Geometry: final body of the model. Coordinates: model frame, mm. Face numbers are marked on the shaded views. A direction names the side the tool comes from. Give positions to 0.01 mm unless a question says otherwise; leave off trailing zeros. Loops run counter-clockwise (first coordinate to the right, second up) from the corner with the lowest first, then second, coordinate; pieces in that order, holes last. Notation, with made-up numbers: (58.5, 20.25) -> (83.5, 20.25) arc R18 cw to (83.5, 38.25) -> close; hole circle Ø9 at (-37, 89.5). An arc over 180 degrees is marked (long way). Answer in a Markdown table with one row per item. Add a question column.
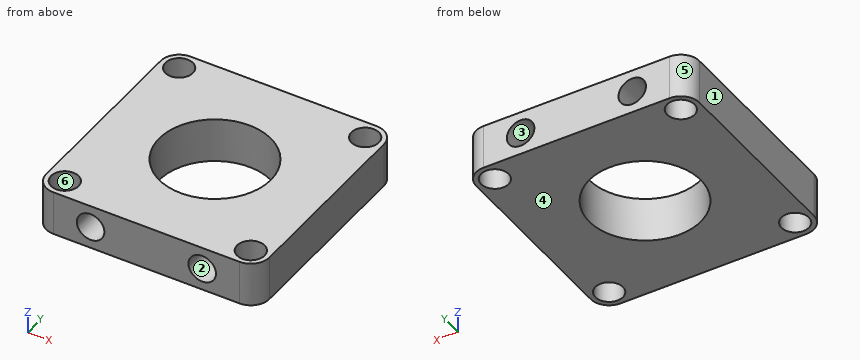
Autodesk Inventor part; units mm, degrees
ref_plane "YZ Plane" through (0, 0, 0) normal (1, 0, 0) x (0, 1, 0)
ref_plane "XZ Plane" through (0, 0, 0) normal (0, 1, 0) x (-1, 0, 0)
ref_plane "XY Plane" through (0, 0, 0) normal (0, 0, 1) x (1, 0, 0)
sketch "Sketch1" plane through (0, 0, 0) normal (0, 0, 1) x (1, 0, 0)
  line L0 (0, 0) -> (38.1, 0)
  line L1 (38.1, 0) -> (38.1, 38.1)
  line L2 (38.1, 38.1) -> (0, 38.1)
  line L3 (0, 38.1) -> (0, 0)
  circle A0 centre (3.175, 34.925) radius 2.3495
  circle A1 centre (34.925, 34.925) radius 2.3495
  circle A2 centre (3.175, 3.175) radius 2.3495
  circle A3 centre (34.925, 3.175) radius 2.3495
  line L4 (0, 19.05) -> (19.05, 19.05)
  circle A4 centre (19.05, 19.05) radius 9.525
  circle A5 centre (19.05, 19.05) radius 6.35
  line L5 (7.4295, 34.925) -> (7.4295, 38.1)
  line L6 (0, 30.6705) -> (3.175, 30.6705)
  arc A6 (3.175, 30.6705) -> (7.4295, 34.925) centre (3.175, 34.925) ccw
  line L7 (5.5245, 34.925) -> (7.4295, 34.925)
  line L8 (3.175, 7.4295) -> (0, 7.4295)
  line L9 (7.4295, 0) -> (7.4295, 3.175)
  arc A7 (7.4295, 3.175) -> (3.175, 7.4295) centre (3.175, 3.175) ccw
  line L10 (30.6705, 3.175) -> (30.6705, 0)
  line L11 (38.1, 7.4295) -> (34.925, 7.4295)
  arc A8 (34.925, 7.4295) -> (30.6705, 3.175) centre (34.925, 3.175) ccw
  line L12 (34.925, 30.6705) -> (38.1, 30.6705)
  line L13 (30.6705, 38.1) -> (30.6705, 34.925)
  arc A9 (30.6705, 34.925) -> (34.925, 30.6705) centre (34.925, 34.925) ccw
  line L14 (0, 7.4295) -> (0, 0)
  line L15 (0, 0) -> (7.4295, 0)
  line L16 (30.6705, 0) -> (38.1, 0)
  line L17 (38.1, 0) -> (38.1, 7.4295)
  line L18 (30.6705, 38.1) -> (38.1, 38.1)
  line L19 (38.1, 38.1) -> (38.1, 30.6705)
  dimension "d2" = 4.699
  dimension "d0" = 38.1
  dimension "d1" = 38.1
  dimension "d5" = 31.75
  dimension "d8" = 31.75
  dimension "d11" = 3.175
  dimension "d12" = 3.175
  dimension "d13" = 19.05
  dimension "d14" = 19.05
  dimension "d15" = 12.7
  dimension "d16" = 3.175
  dimension "d17" = 3.175
  dimension "d18" = 1.905
  dimension "d24" = 360
extrude "Extrusion1" add sketch "Sketch1" along normal blind 7.62 contours L3 L8 A7 L9 L0 | L9 A7 L8 L3 L6 A6 L5 L2 L13 A9 L12 L1 L11 A8 L10 L0 | L10 A8 L11 L1 L0 | L3 L2 L5 A6 L6 | L12 A9 L13 L2 L1
fillet "Fillet1" radius 3.175 4 edges at (0, 38.1, 3.81) (38.1, 38.1, 3.81) (0, 0, 3.81) (38.1, 0, 3.81)
sketch "Sketch2" plane through (3.175, 38.1, 0) normal (0, 1, 0) x (1, 0, 0)
  line L0 (31.75, 0) -> (0, 0)
  line L1 (0, -7.62) -> (31.75, -7.62)
  line L2 (15.875, 0) -> (15.875, -3.81)
  line L3 (15.875, -3.81) -> (25.4, -3.81)
  line L4 (15.875, -3.81) -> (6.35, -3.81)
  circle A0 centre (25.4, -3.81) radius 2.3495
  circle A1 centre (6.35, -3.81) radius 2.3495
  point P0 (-3.175, 0)
  dimension "d29" = 3.81
  dimension "d30" = 9.525
  dimension "d31" = 9.525
  dimension "d32" = 4.699
  dimension "d33" = 4.699
extrude "Extrusion2" cut sketch "Sketch2" against normal blind 7.62
sketch "Sketch3" plane through (3.175, 0, 0) normal (0, -1, 0) x (1, 0, 0)
  line L0 (0, 0) -> (31.75, 0)
  line L1 (15.875, 0) -> (15.875, 3.81)
  line L2 (15.875, 3.81) -> (6.35, 3.81)
  line L3 (15.875, 3.81) -> (25.4, 3.81)
  circle A0 centre (6.35, 3.81) radius 2.3495
  circle A1 centre (25.4, 3.81) radius 2.3495
  point P0 (-3.175, 0)
  dimension "d36" = 3.81
  dimension "d37" = 9.525
  dimension "d38" = 9.525
  dimension "d39" = 4.699
  dimension "d40" = 4.699
extrude "Extrusion3" cut sketch "Sketch3" against normal blind 7.62
thread "Thread1"
thread "Thread2"
thread "Thread3"
thread "Thread4"
thread "Thread5"
thread "Thread6"
thread "Thread7"
thread "Thread8"
equation "\"d16\" = d11"
equation "\"d17\" = d11"
properties part number "Gearbox End Plate 2"
(1) Cut plane B-B on y = 4. Return the cut outline in (x, z) (1 decimal).
(2) Cut plane D-D on z = 3.81. State how many separate pieces and enclosed holes the cut face has, then the cut area to 3 significant figures.
(3) Pin query (flat end, axial travel): pin 1 Ø2.5 at (x, z) = (29, 4) entering from -Y; pin 2 Ø2.5 at (x, z) = (9, 4.5) entering from +Y. Return the tip coordinate at first contact, or that it passes through.
(4) Cut plane A-A on x = 19.05. Return the cut outline in (y, z) (3 decimals).
(5) Draft query along X for the marked faces 4, 5 and 6. Return one class per face: +X half, -X half, draft (parallel to the pull), parting line (faces both ways), or undercut.
(6) Material intervals for line 1 along X through (y, z) = (34.75, 3.81); line 2 along Y through (x, z) = (3, 1.25); line 3 along Y through (x, z) = (33, 5.5), sorted ascending. Write a range as from..to.
(7) Reachability of the marked faces 1, 2 and 3 from +Z, -Z, +X, -X, +Y, -Y: full face, straight path, thin tool, end or side. Return the list, or none.
Answer list:
| question | item | result |
|---|---|---|
| 1 | outline | (0, 0) -> (1, 0) -> (1, 7.6) -> (0, 7.6) -> close; (5.4, 0) -> (32.7, 0) -> (32.7, 7.6) -> (5.4, 7.6) -> close; (37.1, 0) -> (38.1, 0) -> (38.1, 7.6) -> (37.1, 7.6) -> close; hole circle Ø4.7 at (9.5, 3.8); hole circle Ø4.7 at (28.6, 3.8) |
| 2 | separate pieces | 1 |
| 2 | enclosed holes | 5 |
| 2 | area | 945 mm² |
| 3 | pin 1 | stops at y = 7.62 |
| 3 | pin 2 | stops at y = 30.48 |
| 4 | outline | (0, 0) -> (9.525, 0) -> (9.525, 7.62) -> (0, 7.62) -> close; (28.575, 0) -> (38.1, 0) -> (38.1, 7.62) -> (28.575, 7.62) -> close |
| 5 | face 4 | draft |
| 5 | face 5 | -X half |
| 5 | face 6 | undercut |
| 6 | line 1 | x = 0..0.83, 5.52..7.18, 11.87..26.23, 30.92..32.58, 37.27..38.1 |
| 6 | line 2 | y = 0..0.83, 5.52..32.58, 37.27..38.1 |
| 6 | line 3 | y = 0..1.83, 4.52..33.58, 36.27..38.1 |
| 7 | face 1 | +Z, -Z, -X, +Y, -Y |
| 7 | face 2 | -Y |
| 7 | face 3 | +Y |
